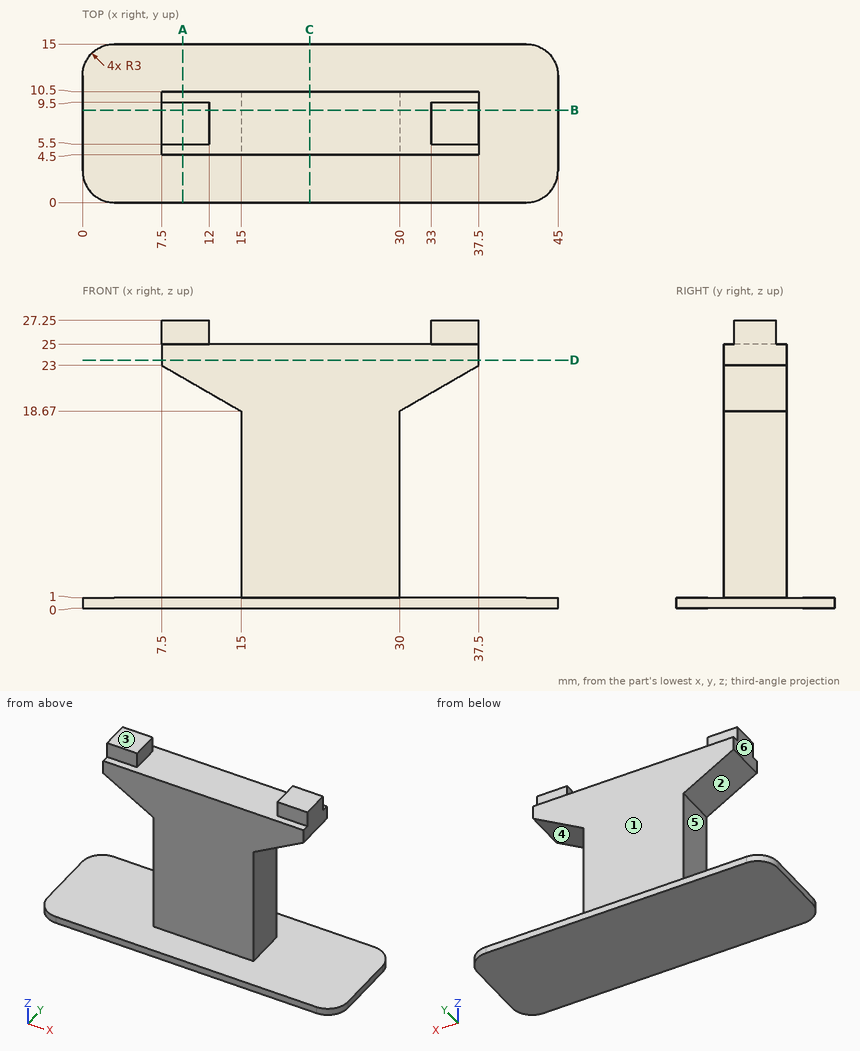
Input: dimensioned drawing with shaded views. Units: mm. Origin: part minimum x, y, z. A direction names the side the tool comes from. Round coordinates to 2 decimals unless told otherwise and drop trailing zeros. Order: outer loops, then holes, each group sorted by start corner. A loop starts at its lowest first (then second) coordinate and runs counter-clockwise, first axis right, second up. Notation, with made-up numbers: (-8.5, 68) -> (5.5, 68) arc R25 cw to (5.5, 99) -> close; hole circle Ø8 at (79, 32). An arc over 180 degrees is marked (long way). One line per item, written item: value. Start each with the question number.
Q1. Material intervals for probe 1 along X at (y, z) = (7.75, 24); probe 2 along Z at (x, y) = (37, 3.5); probe 3 along X at (y, z) = (9, 18.5), sorted ascending.
Q2. Access query for the marked faces 4, 5 and 6. Directions: +Z, -Z, +X, -X, +Y, -Y. A direction counts if a zero-diameter tool reaches every point of the face in a straight line with its end or side. Return the directions, or none.
Q3. Draft query along Z for the marked faces 1, 2 and 3. Return one class per face: pulls with the +Z half, pulls with the -Z half, needs draft (parallel to the pull), parting line crosses it, or undercut.
Q4. Pin query (flat end, axial travel): pin 1 (2 mm diameter, centred on x = 27, z = 9.5, fed in from +Y); pin 2 (0.7 mm diameter, centred on x = 35.5, z = 25.5, fed in from -Y); pin 3 (2.5 mm diameter, centred on y = 8, z = 26.5, fed in from +X). Return the tip coordinate at first contact, or that it passes through.
Q5. Section query C-C (x = 21.5). Return the cut outline in (y, z).
Q6. Section query D-D (z = 23.5). Return the cut outline in (x, y), plus the area to 3 significant figures.
Q7. Section query A-A (x = 9.5). Return the cut outline in (y, z).
Q8. Section query B-B (y = 8.75). Return the cut outline in (x, z), plus the area to 3 significant figures.
Findings below:
1. probe 1: 7.5 to 37.5
1. probe 2: 0 to 1
1. probe 3: 15 to 30
2. face 4: +X, +Y, -Y
2. face 5: -X, +Y, -Y
2. face 6: +Z, -X, +Y, -Y
3. face 1: needs draft
3. face 2: undercut
3. face 3: pulls with the +Z half
4. pin 1: y = 10.5
4. pin 2: y = 5.5
4. pin 3: x = 37.5
5. outline: (0, 0) -> (15, 0) -> (15, 1) -> (10.5, 1) -> (10.5, 25) -> (4.5, 25) -> (4.5, 1) -> (0, 1) -> close
6. outline: (7.5, 4.5) -> (37.5, 4.5) -> (37.5, 10.5) -> (7.5, 10.5) -> close
6. area: 180 mm²
7. outline: (0, 0) -> (15, 0) -> (15, 1) -> (0, 1) -> close; (4.5, 21.85) -> (10.5, 21.85) -> (10.5, 25) -> (9.5, 25) -> (9.5, 27.25) -> (5.5, 27.25) -> (5.5, 25) -> (4.5, 25) -> close
8. outline: (0, 0) -> (45, 0) -> (45, 1) -> (30, 1) -> (30, 18.67) -> (37.5, 23) -> (37.5, 27.25) -> (33, 27.25) -> (33, 25) -> (12, 25) -> (12, 27.25) -> (7.5, 27.25) -> (7.5, 23) -> (15, 18.67) -> (15, 1) -> (0, 1) -> close
8. area: 488 mm²
